Could you check a few things on this drawing? It's one solid part, dimensions in mm from its lowest x, y, z. A direction names the side the tool comes from. Coordinates: 2 decimals unless noted, no trailing zeros. Order: outer loops, then holes, each group sorted by start corner. A loop starts at its lowest first (then second) coordinate and runs counter-clockwise, first axis right, second up. Notation, with made-up numbers: M -28.5,-2 L 17.5,-2 A15 ccw 17.5,18 Z; hole C 14,88 d10. An arc over 180 degrees is marked long. Answer as CSV lines item,"result". Start each with the question number.
1. Will these pins go through, and if not, where does the flat tip stop? pin 1 (0.8 mm diameter, centred on x = 12, z = 40, fed in from -Y); pin 2 (12 mm diameter, centred on x = 10, z = 12.5, fed in from -Y); pin 3 (4 mm diameter, centred on x = 8, y = 2.5, fed in from +Z).
2. On a 3-axis mill with a long thin cutter (end or side, diameter ignored), from which of +Z, -Z, +X, -X, +Y, -Y can I reach the whole of each face in a straight line? I mean the marked faces 1 and 2. Say none if no direction works.
3. If we section it at C-C (z = 39.5): List the corners of the cut face in (x, y) for me, plus the area to 4 significant figures.
4. If we section it at B-B (x = 10.5): List the corners of the cut face in (y, z) for me.
5. I need wall thicknesses on line 1 along Z through (x, y) = (13.5, 3.5); line 2 along Y through (x, z) = (19.25, 37); line 3 along Z through (x, y) = (9.25, 1). Which ranges of each line are inside material? Lowest first, please. Write a range as from..to.
6. If we section it at A-A (y = 4.5): List the corners of the cut face in (x, z) for me.
7. If we section it at D-D (x = 19): List the corners of the cut face in (y, z) for me, plus the area to 3 significant figures.
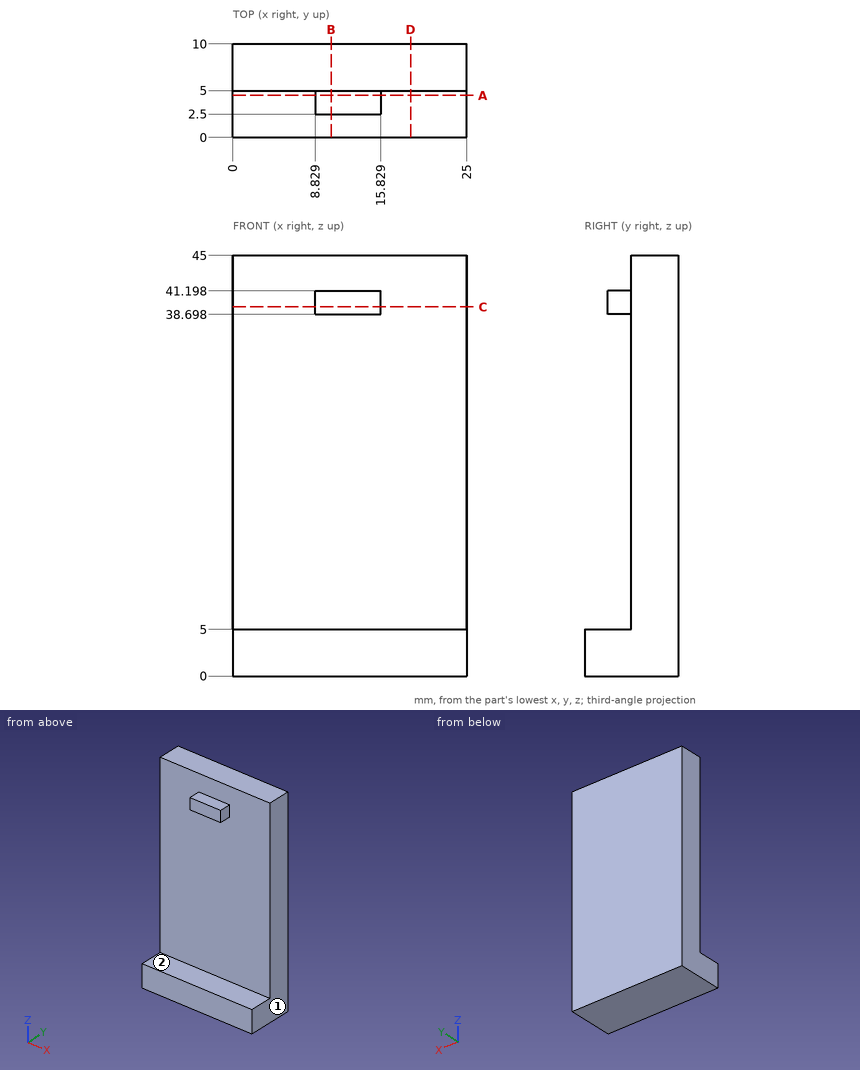
Solved:
1,pin 1,"y = 2.5"
1,pin 2,"y = 5"
1,pin 3,"z = 41.2"
2,face 1,"+Z, -Z, +X, +Y, -Y"
2,face 2,"+X, -X, -Y"
3,outline,"M 0,5 L 8.83,5 L 8.83,2.5 L 15.83,2.5 L 15.83,5 L 25,5 L 25,10 L 0,10 Z"
3,area,"142.5 mm²"
4,outline,"M 0,0 L 10,0 L 10,45 L 5,45 L 5,41.2 L 2.5,41.2 L 2.5,38.7 L 5,38.7 L 5,5 L 0,5 Z"
5,line 1,"0..5, 38.7..41.2"
5,line 2,"5..10"
5,line 3,"0..5"
6,outline,"M 0,0 L 25,0 L 25,5 L 0,5 Z; M 8.83,38.7 L 15.83,38.7 L 15.83,41.2 L 8.83,41.2 Z"
7,outline,"M 0,0 L 10,0 L 10,45 L 5,45 L 5,5 L 0,5 Z"
7,area,"250 mm²"
